```python
from build123d import *

# Parameters (mm, degrees)
SKETCH1_W               = 63
SKETCH1_H               = 45
SKETCH1_R               = 2
SKETCH1_W_2             = 43
SKETCH1_H_2             = 25
BOSS_EXTRUDE1_DEPTH     = 10
SKETCH2_W               = 10
SKETCH2_H               = 20
BOSS_EXTRUDE2_DEPTH     = 76.2
SKETCH3_W               = 10
SKETCH3_H               = 10
BOSS_EXTRUDE3_DEPTH     = 91.6
SKETCH5_W               = 10
SKETCH5_H               = 101.6
BOSS_EXTRUDE4_DEPTH     = 10
CUT_EXTRUDE1_DEPTH      = 158.219909681
CUT_EXTRUDE1_DEPTH_BACK = 158.219909681
SKETCH4_R               = 1.5
FILLET5_R               = 20
FILLET7_R               = 20
FILLET8_R               = 3
FILLET9_START           = 22.5
FILLET9_DEPTH           = 20.0000001
FILLET9_START_2         = 10
FILLET9_2_DEPTH         = 11
FILLET9_3_DEPTH         = 10
SKETCH6_W               = 10
SKETCH6_H               = 20
CUT_EXTRUDE2_DEPTH      = 10
SKETCH7_R               = 1.5
CUT_EXTRUDE3_DEPTH      = 152.539104801


with BuildPart() as part:
    # Sketch1 → Boss-Extrude1 (new body)
    with BuildSketch(Plane(origin=(0, 0, 0), x_dir=(1, 0, 0), z_dir=(0, 1, 0))):
        Rectangle(SKETCH1_W, SKETCH1_H)
        with Locations(Location((-24.75, 5, 0), (0, 0, 270))):
            Circle(SKETCH1_R, mode=Mode.SUBTRACT)
        with Locations(Location((-24.75, -5, 0), (0, 0, 270))):
            Circle(SKETCH1_R, mode=Mode.SUBTRACT)
        with Locations(Location((24.75, 5, 0), (0, 0, 270))):
            Circle(SKETCH1_R, mode=Mode.SUBTRACT)
        with Locations(Location((24.75, -5, 0), (0, 0, 270))):
            Circle(SKETCH1_R, mode=Mode.SUBTRACT)
        Rectangle(SKETCH1_W_2, SKETCH1_H_2, mode=Mode.SUBTRACT)
    extrude(amount=BOSS_EXTRUDE1_DEPTH)

    # Sketch2 → Boss-Extrude2 (add)
    with BuildSketch(Plane.ZY.offset(31.5)):
        with Locations((17.5, 10)):
            Rectangle(SKETCH2_W, SKETCH2_H)
    extrude(amount=BOSS_EXTRUDE2_DEPTH)

    # Sketch3 → Boss-Extrude3 (add)
    with BuildSketch(Plane.XY.offset(22.5)):
        with Locations((-26.5, 5)):
            Rectangle(SKETCH3_W, SKETCH3_H)
    extrude(amount=BOSS_EXTRUDE3_DEPTH)

    # Sketch5 → Boss-Extrude4 (add)
    with BuildSketch(Plane(origin=(0, 10, 0), x_dir=(1, 0, 0), z_dir=(0, 1, 0))):
        with Locations((-26.5, -63.3)):
            Rectangle(SKETCH5_W, SKETCH5_H)
    extrude(amount=BOSS_EXTRUDE4_DEPTH)

    # Sketch4 → Cut-Extrude1 (cut, two sides: drawn at the far end of the back side and taken through both)
    with BuildSketch(Plane(origin=(0, 10, 0), x_dir=(1, 0, 0), z_dir=(0, 1, 0)).offset(-CUT_EXTRUDE1_DEPTH_BACK)):
        with BuildLine():
            ThreePointArc((-91.2, -17.5), (-92.7, -16), (-94.2, -17.5))
            Line((-94.2, -17.5), (-91.2, -17.5))
        make_face()
        with BuildLine():
            Line((-91.2, -17.5), (-94.2, -17.5))
            ThreePointArc((-94.2, -17.5), (-92.7, -19), (-91.2, -17.5))
        make_face()
        with Locations(Location((-66.5, -17.5, 0), (0, 0, 270))):
            Circle(SKETCH4_R)
        with Locations(Location((-36.5, -17.5, 0), (0, 0, 270))):
            Circle(SKETCH4_R)
    extrude(amount=CUT_EXTRUDE1_DEPTH + CUT_EXTRUDE1_DEPTH_BACK, mode=Mode.SUBTRACT)

    # Fillet5
    fillet5_edges = [part.edges().sort_by_distance(p)[0] for p in [
        (-31.5, 5, 12.5),
        (-31.5, 10, 22.5),
    ]]
    fillet(fillet5_edges, radius=FILLET5_R)

    # Fillet7
    # the kernel refuses this fillet: 20 mm, written as the material it adds along each edge
    with BuildSketch(Plane(origin=(-21.5, 10, 12.5), x_dir=(1, 0, 0), z_dir=(0, 0, 1))) as fillet7_piece_1:
        with BuildLine():
            CenterArc((17.320508076, 20), FILLET7_R, 210, 60)
            Line((0, 10), (-0.346410162, 9.8))
            ThreePointArc((-0.346410162, 9.8), (-0.4, 5), (-0.4, 0))
            Line((-0.4, 0), (0, -0.4))
            Line((0, -0.4), (17.320508076, -0.4))
            Line((17.320508076, -0.4), (17.320508076, 0))
        make_face()
    extrude(amount=10)

    # Fillet8
    fillet8_edges = [part.edges().sort_by_distance(p)[0] for p in [
        (-36.5, 10, 12.5),
    ]]
    fillet(fillet8_edges, radius=FILLET8_R)

    # Fillet9: read off the stored shape, not the designer's step
    # Fillet9 outline → Fillet9 (add)
    with BuildSketch(Plane.XY.offset(FILLET9_START)):
        with BuildLine():
            Line((-21.5, 10), (-4.179491924, 10))
            ThreePointArc((-4.179491924, 10), (-14.179495423, 12.679493944), (-21.50000404, 20.000006998))
            Line((-21.50000404, 20.000006998), (-21.5, 10))
        make_face()
    extrude(amount=FILLET9_DEPTH)

    # Fillet9 2 outline → Fillet9 2 (cut)
    with BuildSketch(Plane(origin=(0, 0, 0), x_dir=(1, 0, 0), z_dir=(0, 1, 0)).offset(FILLET9_START_2)):
        with BuildLine():
            ThreePointArc((-1.5, -22.5), (-15.642135624, -28.357864376), (-21.5, -42.5))
            Line((-21.5, -42.5), (0, -42.5000001))
            Line((0, -42.5000001), (0, -22.5))
            Line((0, -22.5), (-1.5, -22.5))
        make_face()
    extrude(amount=FILLET9_2_DEPTH, mode=Mode.SUBTRACT)

    # Fillet9 3 outline → Fillet9 3 (add)
    with BuildSketch(Plane(origin=(0, 0, 0), x_dir=(1, 0, 0), z_dir=(0, 1, 0))):
        with BuildLine():
            Line((-21.5, -22.5), (-21.5, -42.5))
            ThreePointArc((-21.5, -42.5), (-15.642135624, -28.357864376), (-1.5, -22.5))
            Line((-1.5, -22.5), (-21.5, -22.5))
        make_face()
    extrude(amount=FILLET9_3_DEPTH)

    # Sketch6 → Cut-Extrude2 (cut)
    with BuildSketch(Plane.ZY.offset(107.7)):
        with Locations((17.5, 10)):
            Rectangle(SKETCH6_W, SKETCH6_H)
    extrude(amount=-CUT_EXTRUDE2_DEPTH, mode=Mode.SUBTRACT)

    # Sketch7 → Cut-Extrude3 (cut, through all)
    with BuildSketch(Plane(origin=(0, 0, 0), x_dir=(-1, 0, 0), z_dir=(0, -1, 0))):
        with Locations(Location((26.5, -54.1, 0), (0, 0, 90))):
            Circle(SKETCH7_R)
        with Locations(Location((26.5, -94.1, 0), (0, 0, 90))):
            Circle(SKETCH7_R)
        with Locations(Location((26.5, -74.1, 0), (0, 0, 90))):
            Circle(SKETCH7_R)
        with Locations(Location((26.5, -104.1, 0), (0, 0, 90))):
            Circle(SKETCH7_R)
    extrude(amount=-CUT_EXTRUDE3_DEPTH, mode=Mode.SUBTRACT)


solid = part.part
```
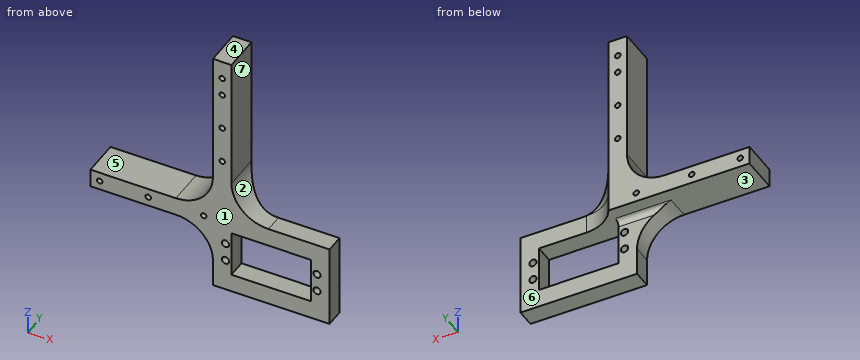
Input: part model. Units: mm. Frame: model coordinates. Face numbers are marked on the shaded views. A direction names the side the tool comes from. Coordinates: 2 decimals unless noted, no trailing zeros. Loops run counter-clockwise (first coordinate to the right, second up) from the corner with the lowest first, then second, coordinate; pieces in that order, holes last. Notation, with made-up numbers: M 84.5,31.5 L 115.5,31.5 A23 cw 115.5,53.5 Z; hole C -23.75,89.25 d9. An arc over 180 degrees is marked long. Answer in a Markdown table with one row per item.
1. First-contact query: pin 1 (4.5 mm diameter, centred on x = 24.75, z = -5, fed in from +Y); pin 2 (10 mm diameter, centred on y = 8, z = 64.5, fed in from -X); pin 3 (5 mm diameter, centred on y = 8.5, z = 54, fed in from +X). Flat tips, straight axial feed; report the tip coordinate or a pass-through.
Response:
| item | result |
|---|---|
| pin 1 | stops at y = 10 |
| pin 2 | stops at x = -31.5 |
| pin 3 | stops at x = -21.5 |
2. Draft query along Z for the marked faces 1, 2 and 3. Return one class per face: pulls with the +Z half, pulls with the -Z half, needs draft (parallel to the pull), parting line crosses it, or undercut.
Response:
| item | result |
|---|---|
| face 1 | needs draft |
| face 2 | pulls with the +Z half |
| face 3 | undercut |
3. Material intervals for line 1 (Z direction, x = 12.5, y = 1.75); line 2 (Z direction, x = -26, y = 11.25); line 3 (X direction, y = 10, z = 54), sorted ascending.
Response:
| item | result |
|---|---|
| line 1 | z = -22.5 to -12.5, 12.5 to 22.5 |
| line 2 | z = 11.94 to 52.69, 55.51 to 72.69, 75.51 to 92.69, 95.51 to 102.69, 105.51 to 114.1 |
| line 3 | x = -31.5 to -28, -25 to -21.5 |
4. Section A-A, the plane y = 5.5. Count the separate pieces of the cut face and the enclosed holes in it, then the cut area to 3 significant figures.
Response:
| item | result |
|---|---|
| separate pieces | 1 |
| enclosed holes | 12 |
| area | 3,500 mm2 |
5. Section C-C, the plane z = 5. Output: boundary loops of the cut face in (x, y).
Response:
| item | result |
|---|---|
| outline | M -35.89,0 L -26.75,0 L -26.75,10 L -35.89,10 Z; M -22.75,0 L -21.5,0 L -21.5,10 L -22.75,10 Z; M 21.5,0 L 22.75,0 L 22.75,10 L 21.5,10 Z; M 26.75,0 L 31.5,0 L 31.5,10 L 26.75,10 Z |
6. Reachability of the marked faces 4, 5, 6 and 7 from +Z, -Z, +X, -X, +Y, -Y: full face, straight path, thin tool, end or side. Return the list, or none.
Response:
| item | result |
|---|---|
| face 4 | +Z, +X, -X, +Y, -Y |
| face 5 | +Z, -X, +Y, -Y |
| face 6 | -Z, +X, +Y |
| face 7 | +Z, +X, +Y, -Y |
7. Section B-B, the plane x = 7.5. Output: boundary loops of the cut face in (y, z), then the cut area to 3 significant figures.
Response:
| item | result |
|---|---|
| outline | M 0,-22.5 L 10,-22.5 L 10,-12.5 L 0,-12.5 Z; M 0,12.5 L 10,12.5 L 10,22.5 L 0,22.5 Z |
| area | 200 mm2 |
